```python
from build123d import *

# Parameters (mm, degrees)
PAD_DEPTH       = 17.5
POCKET_DEPTH    = 5
POCKET001_DEPTH = 5
SKETCH003_R     = 1.5
POCKET002_DEPTH = 3.001
SKETCH005_R     = 8.354384
SKETCH005_R_2   = 5.120413
SKETCH005_R_3   = 2.670225
POCKET004_DEPTH = 30.001
FILLET_R        = 2


with BuildPart() as part:
    # Sketch → Pad (new body, symmetric)
    with BuildSketch(Plane.XY):
        Polygon((-1.824811, 2.017518), (-1.824811, -26.893557), (60.175189, -26.893557), align=None)
    extrude(amount=PAD_DEPTH, both=True)

    # Sketch001 → Pocket (cut)
    with BuildSketch(Plane.XY.offset(17.5)):
        Polygon((-1.824811, 2.017518), (-1.824811, -23.893557), (53.741669, -23.893557), align=None)
    extrude(amount=-POCKET_DEPTH, mode=Mode.SUBTRACT)

    # Sketch002 → Pocket001 (cut)
    with BuildSketch(Plane(origin=(0, 0, -17.5), x_dir=(1, 0, 0), z_dir=(0, 0, -1))):
        Polygon((53.741669, 23.893557), (-1.824811, 23.893557), (-1.824811, -2.017518), align=None)
    extrude(amount=-POCKET001_DEPTH, mode=Mode.SUBTRACT)

    # Sketch003 → Pocket002 (cut, through all)
    with BuildSketch(Plane(origin=(0, -23.893557, 0), x_dir=(-1, 0, 0), z_dir=(0, 1, 0))):
        with Locations((-50.175189, 14.5)):
            Circle(SKETCH003_R)
        with Locations((-3.175189, 14.5)):
            Circle(SKETCH003_R)
        with Locations((-50.175189, -14.5)):
            Circle(SKETCH003_R)
        with Locations((-3.175189, -14.5)):
            Circle(SKETCH003_R)
    extrude(amount=-POCKET002_DEPTH, mode=Mode.SUBTRACT)

    # Sketch005 → Pocket004 (cut, through all)
    with BuildSketch(Plane.XY.offset(12.5)):
        with Locations((8.700624, -14.118617)):
            Circle(SKETCH005_R)
        with Locations((26.303152, -18.020678)):
            Circle(SKETCH005_R_2)
        with Locations((38.438648, -20.737577)):
            Circle(SKETCH005_R_3)
    extrude(amount=-POCKET004_DEPTH, mode=Mode.SUBTRACT)

    # Fillet
    fillet_edges = [part.edges().sort_by_distance(p)[0] for p in [
        (25.958429, -23.893557, -17.5),
    ]]
    fillet(fillet_edges, radius=FILLET_R)


solid = part.part
```
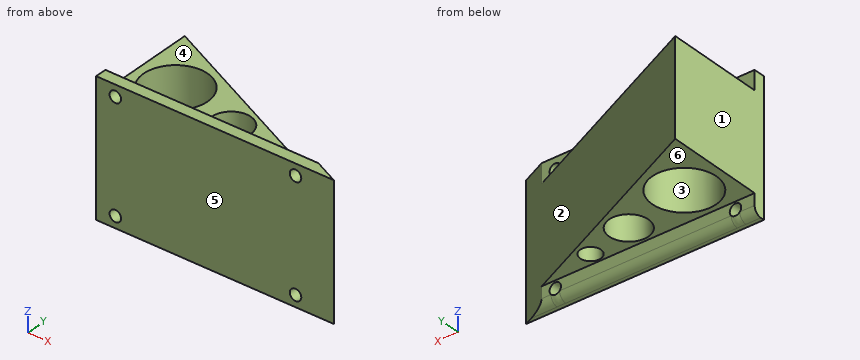
Model file for the job. Use its own axes, mm. Face numbers are marked on the shaded views. A direction names the side the tool comes from. Coordinates: 2 decimals unless noted, no trailing zeros. Write each loop counter-clockwise with the first axis right and the second up, starting at its lowest first coordinate (ties: lowest second). Pieces come first, ordered by that corner, then holes. Notation, with made-up numbers: (11, 42) - (51, 42) arc R21 ccw to (51, 64) - close; hole circle Ø6 at (16, 28). An arc over 180 degrees is marked (long way). One line per question, with ' | ' between items. Start each with the question number.
Q1. Cut at D-D, the plane y = -7.5. List the corners of the cut face in (x, z), then the cut area to 3 significant figures.
Q2. Cut at B-B, the plane x = 12. List the corners of the cut face in (y, z), then the cut area to 3 significant figures.
Q3. Pull direction Y, two halves, no side cores. Call the marked faces 1, 2 and 3: pulls with the +Y half, pulls with the -Y half, needs draft (parallel to the pull), parting line crosses it, or undercut.
Q4. Cut at A-A, the plane z = -14.5. List the corners of the cut face in (x, y), then the cut area to 3 significant figures.
Q5. Cut at C-C, the plane y = -15. List the corners of the cut face in (x, z), then the cut area to 3 significant figures.
Q6. Drill centre lines: line 1 (X direction, y = -18, z = -8); line 2 (X direction, y = -14.5, z = -11); line 3 (Y direction, x = 36.5, z = -14.5). Where is each one in solid material? Low to high. Write a range as [from, to].
Q7. Pin check, flat tips, straight feed: pin 1 (13.5 mm diameter, centred on x = 8.7, y = -14.12, fed in from -Z); pin 2 (6 mm diameter, centred on y = -18, z = 12.5, fed in from +X); pin 3 (5.5 mm diameter, centred on x = 30.5, z = 14, fed in from +Y); pin 4 (10 mm diameter, centred on y = -24, z = -12, fed in from +X). Stop position of each tip, or through.
Q8. 3-axis set-ups, long thin cutter, end or side, ignore diameter. For the marked faces 4, 5 and 6: which of +Z, -Z, +X, -X, +Y, -Y reach the whole face in a straight line?
Answer below:
1) outline: (-1.82, -12.5) - (3.6, -12.5) - (3.6, 12.5) - (-1.82, 12.5) - close; (13.8, -12.5) - (18.59, -12.5) - (18.59, 12.5) - (13.8, 12.5) - close | area: 255 mm^2
2) outline: (-26.89, -17.5) - (-25.89, -17.5) arc R2 ccw to (-23.89, -15.5) - (-23.89, -12.5) - (-21.79, -12.5) - (-21.79, 12.5) - (-23.89, 12.5) - (-23.89, 17.5) - (-26.89, 17.5) - close; (-6.44, -12.5) - (-4.43, -12.5) - (-4.43, 12.5) - (-6.44, 12.5) - close | area: 207 mm^2
3) face 1: needs draft | face 2: pulls with the +Y half | face 3: undercut
4) outline: (-1.82, -26.89) - (1.68, -26.89) - (1.68, -23.89) - (-1.82, -23.89) - close; (4.68, -26.89) - (48.68, -26.89) - (48.68, -23.89) - (4.68, -23.89) - close; (51.68, -26.89) - (60.18, -26.89) - (53.74, -23.89) - (51.68, -23.89) - close | area: 158 mm^2
5) outline: (-1.82, -12.5) - (0.39, -12.5) - (0.39, 12.5) - (-1.82, 12.5) - close; (17.01, -12.5) - (22.17, -12.5) - (22.17, 12.5) - (17.01, 12.5) - close; (30.44, -12.5) - (34.67, -12.5) - (34.67, 12.5) - (30.44, 12.5) - close | area: 290 mm^2
6) line 1: [-1.82, 1.3], [16.1, 21.18], [31.42, 41.1] | line 2: [-1.82, 0.35], [17.05, 22.59], [30.02, 33.6] | line 3: [-26.89, -23.89]
7) pin 1: through | pin 2: x = 47.54 | pin 3: y = -11.98 | pin 4: x = 60.18
8) face 4: +Z, +X, -X, +Y | face 5: +Z, -Z, +X, -X, -Y | face 6: -Z, +X, -X, +Y
